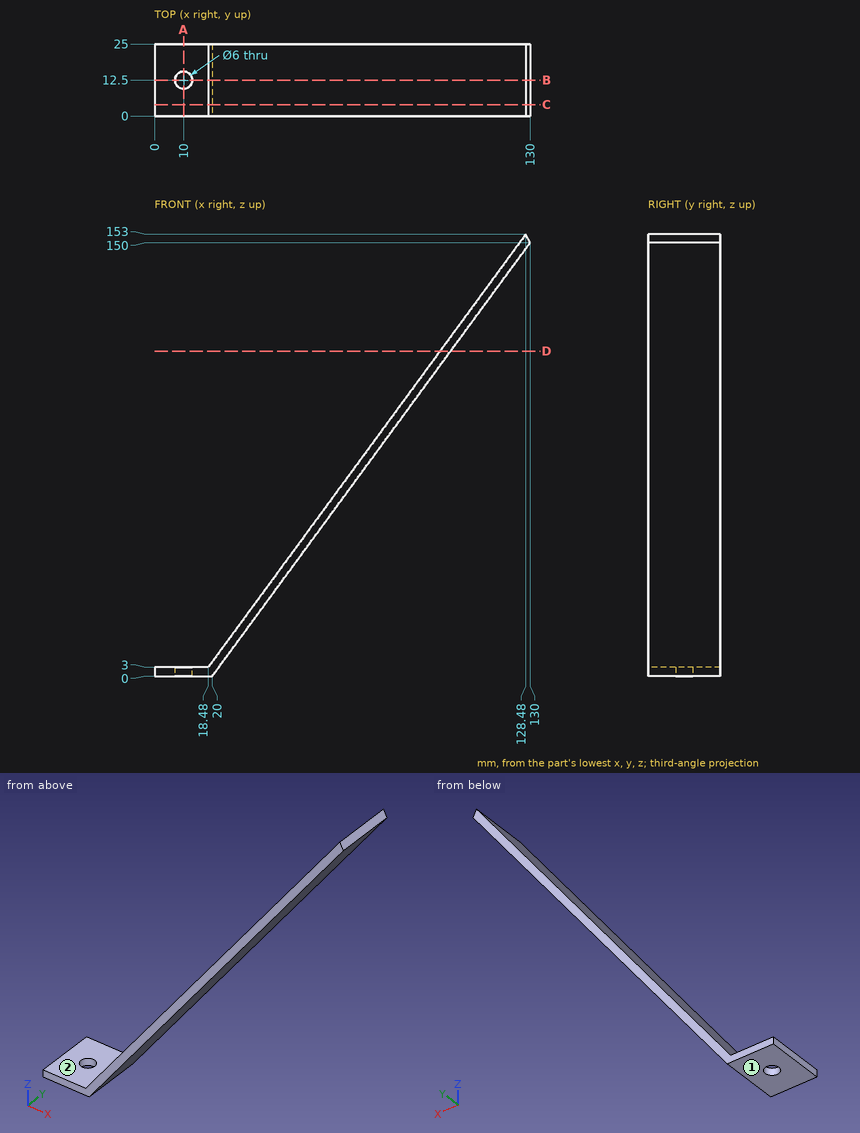
For this review, use the dimensioned drawing (mm, ordinates from the lowest corner) and the shaded views. A direction names the side the tool comes from. Give positions to 0.01 mm unless a question says otherwise; leave off trailing zeros. Loops run counter-clockwise (first coordinate to the right, second up) from the corner with the lowest first, then second, coordinate; pieces in that order, holes last. Notation, with made-up numbers: (12.5, 66.25) - (38.5, 66.25) arc R27 ccw to (38.5, 102.25) - close; hole circle Ø9 at (54.5, -8). An arc over 180 degrees is marked (long way). Write each question's results on one line, items separated by ' | '.
(1) Take a section at A-A (x = 10). Give the boundary of the cut face in (y, z).
Conclusion:
outline: (0, 0) - (9.5, 0) - (9.5, 3) - (0, 3) - close; (15.5, 0) - (25, 0) - (25, 3) - (15.5, 3) - close
(2) For pin 1 Ø5 at (x, y) = (90, 14) entering from -Z (1 decimal); pin 2 Ø9 at (x, y) = (7.5, 12) entering from +Z; pin 3 Ø8 at (y, z) = (8, 22.5) entering from -X, all flat-tipped, find the tip position at first contact; note any pin that passes through.
Conclusion:
pin 1: z = 92 | pin 2: z = 3 | pin 3: x = 29.85
(3) For the marked faces 1 and 2, list the 3-axis set-ups (+Z, -Z, +X, -X, +Y, -Y) from which the entire face can be reached by the end or side of a thin tool; tool diameter is ignored.
Conclusion:
face 1: -Z, +X, -X, +Y, -Y | face 2: +Z, -X, +Y, -Y
(4) For line 1 along Y through (x, z) = (10, 2.05); line 2 along Z through (x, y) = (11.5, 1); line 3 along X through (y, z) = (12.5, 1.6), list the stretches that pass through material, from the lowest coordinate up.
Conclusion:
line 1: 0 to 9.5, 15.5 to 25 | line 2: 0 to 3 | line 3: 0 to 7, 13 to 21.17
(5) Take a section at D-D (z = 112.5). Give the boundary of the cut face in (x, y).
Conclusion:
outline: (98.78, 0) - (102.5, 0) - (102.5, 25) - (98.78, 25) - close
(6) Take a section at C-C (y = 4). Give the boundary of the cut face in (x, z).
Conclusion:
outline: (0, 0) - (20, 0) - (130, 150) - (128.48, 153) - (18.48, 3) - (0, 3) - close
(7) Take a section at B-B (y = 12.5). Give the boundary of the cut face in (x, z).
Conclusion:
outline: (0, 0) - (7, 0) - (7, 3) - (0, 3) - close; (13, 0) - (20, 0) - (130, 150) - (128.48, 153) - (18.48, 3) - (13, 3) - close
